Check sheet for the modelled part. Datum: model origin and axes. Units: mm. Face numbers are marked on the shaded views. A direction names the side the tool comes from. Round coordinates to 2 decimals unless told otherwise and drop trailing zeros. Order: outer loops, then holes, each group sorted by start corner. A loop starts at its lowest first (then second) coordinate and runs counter-clockwise, first axis right, second up. Notation, with made-up numbers: (-36.75, 49.5) -> (22.25, 49.5) arc R22 ccw to (22.25, 74.5) -> close; hole circle Ø11 at (78, 49). An arc over 180 degrees is marked (long way). Use CSV: the item, a comma, the result in double quotes.
Autodesk Inventor part; units mm, degrees
ref_plane "YZ Plane" through (0, 0, 0) normal (1, 0, 0) x (0, 1, 0)
ref_plane "XZ Plane" through (0, 0, 0) normal (0, 1, 0) x (-1, 0, 0)
ref_plane "XY Plane" through (0, 0, 0) normal (0, 0, 1) x (1, 0, 0)
sketch "スケッチ1" plane through (0, 0, 0) normal (0, 1, 0) x (-1, 0, 0)
  line L0 (0, 6.75) -> (-13.5, 6.75) construction
  line L1 (-13.5, 6.75) -> (-13.5, -6.75) construction
  line L2 (-13.5, -6.75) -> (0, -6.75) construction
  line L3 (0, -6.75) -> (0, 6.75) construction
  circle A0 centre (-8, 0) radius 6.5
  line L4 (0, 8.5) -> (-25, 8.5)
  line L5 (-25, 8.5) -> (-25, -8.5)
  line L6 (-25, -8.5) -> (0, -8.5)
  line L7 (0, -8.5) -> (0, 8.5)
  line L8 (-25, 8.5) -> (-27.8, 8.5)
  line L9 (-27.8, 8.5) -> (-27.8, -8.5)
  line L10 (-27.8, -8.5) -> (-25, -8.5)
  line L11 (-25, -8.5) -> (-25, 8.5)
  line L12 (0, 6.5) -> (-8, 6.5)
  line L13 (0, -6.5) -> (-8, -6.5)
  point P0 (0, 0)
  point P1 (0, 0)
  dimension "d0" = 13.5
  dimension "d1" = 13.5
  dimension "d2" = 8
  dimension "d3" = 13
  dimension "d4" = 17
  dimension "d5" = 25
  dimension "d6" = 2.8
extrude "押し出し1" add sketch "スケッチ1" along normal blind 3 contours A0 L13 L7 L6 L5 L4 L12
hole "穴1" at (13.5, 0, -6.75) at (13.5, 0, 6.75) direction (0, 1, 0) diameter 1.6 end through all
sketch "スケッチ2" plane through (0, 0, 8.5) normal (0, 0, 1) x (1, 0, 0)
  line L0 (25, 0) -> (25, 3)
  line L1 (0, 3) -> (25, 3)
  line L2 (25, 0) -> (28, 0)
  line L3 (28, 0) -> (28, 11) construction
  line L4 (28, 11) -> (25, 11)
  line L5 (25, 11) -> (25, 0)
  circle A0 centre (28.1, 5.5) radius 1.1
  arc A1 (30.6287, 7.2932) -> (30.6287, 3.7068) centre (28.1, 5.5) ccw construction
  line L6 (28, 11) -> (30.6287, 7.2932)
  line L7 (28, 0) -> (30.6287, 3.7068)
  arc A2 (30.6287, 3.7068) -> (30.6287, 7.2932) centre (28.1, 5.5) ccw
  dimension "d9" = 2.2
  dimension "d10" = 3
  dimension "d12" = 8
  dimension "d13" = 6.2
extrude "押し出し2" add sketch "スケッチ2" against normal up to surface (17 mm away)
fillet "フィレット1" radius 2 1 edges at (25, 3, 0)
mirror "ミラー1" about plane through (0, 0, -8.5) normal (-1, 0, 0) of "押し出し1", "穴1", "押し出し2", "フィレット1"
properties part number "Ultrasonic_holder"
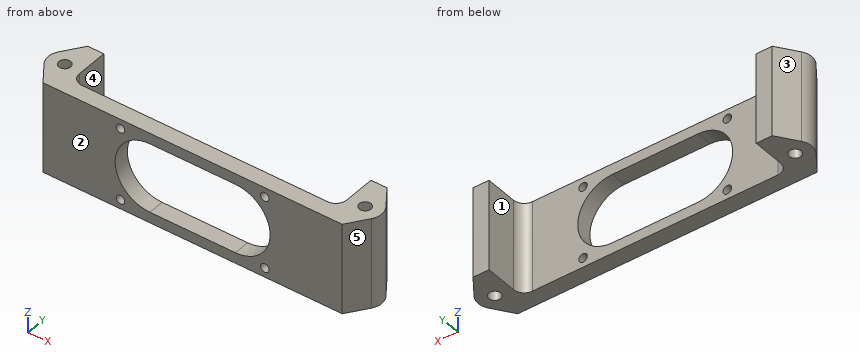
Q1. Access from +Z, -Z, +X, -X, +Y, -Y to the whole of each face (thin tool, end or side, straight path). Record for the marked faces 4 and 5.
Result sheet:
face 4,"+Z, -Z, +Y"
face 5,"+Z, -Z, +X, -Y"
Q2. Scan lines: L1, parallel to X at y = 6, z = 3; L2, parallel to X at y = 4.75, z = 2; L3, parallel to Z at x = 13.5, y = 2. Record each from-to range of solid material in increasing order.
Result sheet:
L1,"x = -31.16 to -29.08, -27.12 to -25, 25 to 27.12, 29.08 to 31.16"
L2,"x = -31.11 to -28.9, -27.3 to -24.98, 24.98 to 27.3, 28.9 to 31.11"
L3,"z = -8.5 to -7.55, -5.95 to -3.46, 3.46 to 5.95, 7.55 to 8.5"
Q3. Mould release check, pull along X, two halves, no side actions. Record for the marked faces 1, 2 and 3: pulls with the +X half, pulls with the -X half, needs draft (parallel to the pull), parting line crosses it, or undercut.
Result sheet:
face 1,"undercut"
face 2,"needs draft"
face 3,"pulls with the -X half"
Q4. Sectioned sample at B-B, the plane x = -3. Enter the section's corners in (y, z).
Result sheet:
outline,"(0, -8.5) -> (3, -8.5) -> (3, -6.5) -> (0, -6.5) -> close; (0, 6.5) -> (3, 6.5) -> (3, 8.5) -> (0, 8.5) -> close"
Q5. Sectioned sample at D-D, the plane y = 9. Enter the section's corners in (x, z), then the cut area to 3 significant figures.
Result sheet:
outline,"(-29.42, -8.5) -> (-25, -8.5) -> (-25, 8.5) -> (-29.42, 8.5) -> close; (25, -8.5) -> (29.42, -8.5) -> (29.42, 8.5) -> (25, 8.5) -> close"
area,"150 mm^2"
Q6. Go/stop test with flat-tipped pins: pin 1 (4 mm diameter, centred on x = -15, y = 6.5, fed in from -Z); pin 2 (4 mm diameter, centred on x = 11.5, z = 6, fed in from +Y); pin 3 (5 mm diameter, centred on y = 9, z = 2.5, fed in from +X). Record where each tip stops, or that it passes through.
Result sheet:
pin 1,"passes through"
pin 2,"stops at y = 3"
pin 3,"stops at x = 31.03"
Q7. Sectioned sample at A-A, the plane z = 0. Enter the section's corners in (x, y), then the cut area to 3 significant figures.
Result sheet:
outline,"(-30.63, 3.71) -> (-28, 0) -> (-14.5, 0) -> (-14.5, 3) -> (-23, 3) arc R2 cw to (-25, 5) -> (-25, 11) -> (-28, 11) -> (-30.63, 7.29) arc R3.1 ccw to start; (14.5, 0) -> (28, 0) -> (30.63, 3.71) arc R3.1 ccw to (30.63, 7.29) -> (28, 11) -> (25, 11) -> (25, 5) arc R2 cw to (23, 3) -> (14.5, 3) -> close; hole circle Ø2.2 at (-28.1, 5.5); hole circle Ø2.2 at (28.1, 5.5)"
area,"164 mm^2"
Q8. Sectioned sample at C-C, the plane x = -13.5. Enter the section's corners in (y, z).
Result sheet:
outline,"(0, -8.5) -> (3, -8.5) -> (3, -7.55) -> (0, -7.55) -> close; (0, -5.95) -> (3, -5.95) -> (3, -3.46) -> (0, -3.46) -> close; (0, 3.46) -> (3, 3.46) -> (3, 5.95) -> (0, 5.95) -> close; (0, 7.55) -> (3, 7.55) -> (3, 8.5) -> (0, 8.5) -> close"
